Work out the finished part from the listing and answer in its coordinate system (mm). A direction names the side the tool comes from. Give positions to 0.01 mm unless a question says otherwise; leave off trailing zeros. Answer in a Markdown table with one row per item. Add a question column.
from build123d import *

# Parameters (mm, degrees)
BOSS_EXTRUDE1_DEPTH = 62
FILLET1_R           = 3
SKETCH2_R           = 4
CUT_EXTRUDE1_DEPTH  = 20


with BuildPart() as part:
    # Sketch1 → Boss-Extrude1 (new body)
    with BuildSketch(Plane(origin=(0, 0, 0), x_dir=(0, 0, -1), z_dir=(1, 0, 0))):
        with BuildLine():
            Line((-43.5, 0), (43.5, 0))
            ThreePointArc((43.5, 0), (47.853804482, 14.177339776), (47.362560683, 29))
            ThreePointArc((47.362560683, 29), (-0.343872677, 30.041597997), (-47.379193576, 22))
            ThreePointArc((-47.379193576, 22), (-47.006596643, 10.723695647), (-43.5, 0))
        make_face()
    extrude(amount=BOSS_EXTRUDE1_DEPTH)

    # Fillet1
    fillet1_edges = [part.edges().sort_by_distance(p)[0] for p in [
        (62, 14.177339776, -47.853804482),
        (62, 30.041597997, 0.343872677),
        (62, 10.723695647, 47.006596643),
        (0, 30.041597997, 0.343872677),
        (0, 14.177339776, -47.853804482),
        (0, 0, 0),
        (0, 10.723695647, 47.006596643),
        (62, 0, 0),
        (31, 22, 47.379193576),
        (31, 29, -47.362560683),
        (31, 0, -43.5),
        (31, 0, 43.5),
    ]]
    fillet(fillet1_edges, radius=FILLET1_R)

    # Sketch2 → Cut-Extrude1 (cut)
    with BuildSketch(Plane.XZ):
        with Locations((11, 5.614286523)):
            Circle(SKETCH2_R)
        with BuildLine():
            ThreePointArc((15, 5.614286523), (11, 1.614286523), (7, 5.614286523))
            Line((7, 5.614286523), (7, -2.442860068))
            ThreePointArc((7, -2.442860068), (11, 1.557139932), (15, -2.442860068))
            Line((15, -2.442860068), (15, 5.614286523))
        make_face()
        with BuildLine():
            ThreePointArc((15, -2.442860068), (11, 1.557139932), (7, -2.442860068))
            Line((7, -2.442860068), (15, -2.442860068))
        make_face()
        with BuildLine():
            Line((15, -2.442860068), (7, -2.442860068))
            ThreePointArc((7, -2.442860068), (11, -6.442860068), (15, -2.442860068))
        make_face()
        with Locations((51, -2.442860068)):
            Circle(SKETCH2_R)
        with BuildLine():
            Line((47, 5.614286523), (47, -2.442860068))
            ThreePointArc((47, -2.442860068), (51, 1.557139932), (55, -2.442860068))
            Line((55, -2.442860068), (55, 5.614286523))
            ThreePointArc((55, 5.614286523), (51, 1.614286523), (47, 5.614286523))
        make_face()
        with Locations((51, 5.614286523)):
            Circle(SKETCH2_R)
    extrude(amount=-CUT_EXTRUDE1_DEPTH, mode=Mode.SUBTRACT)


solid = part.part
(1) Which of the six approach directions +Z, -Z, +X, -X, +Y, -Y give full straight-line access (tool end or side, diameter ignored) to faces 5 (the face through (10.91, 9.86, -6.44)), 6 (the face through (31.39, 0.48, 43.21))?
(2) The mould has two halves that part along Z. Classify faces 1 (the face through (61.1, 0.86, -0.59)), 2 (the face through (51, 20, 2)), 3 (the face through (50.91, 9.86, -6.44)), 4 (the face through (30.608, 30.083, -0.228)): pulls with the +Z half, pulls with the -Z half, needs draft (parallel to the pull), parting line crosses it, or undercut.
(3) Section A-A, the plane y = 5 is taken. State how many separate pieces and enclosed holes the cut face has, and give its area (3 significant figures).
(4) Each of these flat-tipped pins is pushed along its axis until it touches: P1, Ø5, axis at x = 25, y = 11.5, coming from the +Z side; P2, Ø1, axis at x = 20, y = 10, coming from the -Z side; P3, Ø2.5, axis at x = 51, z = 3.5, coming from the -Y side. Where does it stop, or does it pass through?
(5) Consider line 1 along X through (y, z) = (9, -4); line 2 along Z through (x, y) = (49, 2.5); line 3 along Y through (x, z) = (48, -18). Determine where each line is inside the solid, lowest interval first. Write a range as from..to.
Numbers:
| question | item | result |
|---|---|---|
| 1 | face 5 | -Y |
| 1 | face 6 | +Z, +X, -X, -Y |
| 2 | face 1 | needs draft |
| 2 | face 2 | undercut |
| 2 | face 3 | undercut |
| 2 | face 4 | parting line crosses it |
| 3 | separate pieces | 1 |
| 3 | enclosed holes | 2 |
| 3 | area | 5,420 mm² |
| 4 | P1 | stops at z = 47.45 |
| 4 | P2 | stops at z = -47.21 |
| 4 | P3 | stops at y = 20 |
| 5 | line 1 | x = 0..7.32, 14.68..47.32, 54.68..62 |
| 5 | line 2 | z = -44.66..-5.91, 9.08..44.63 |
| 5 | line 3 | y = 0..30.72 |
